Could you check a few things on this model? Use its own coordinates, in mm. Face numbers are marked on the shaded views. A direction names the side the tool comes from. Round coordinates to 2 decimals unless told otherwise and drop trailing zeros. Write each loop counter-clockwise with the first axis right and the second up, starting at its lowest first coordinate (ties: lowest second). Pieces come first, ordered by that corner, then holes. Notation, with made-up numbers: M 52.5,50.25 L 109.5,50.25 A24 ccw 109.5,75.25 Z; hole C 86.5,71.5 d9. An arc over 180 degrees is marked long. One line per item, written item: value. Start each with the question number.
(1) I want a section at A-A on x = 0. Please give me the cut outline in (y, z), and give its area (3 significant figures).
(2) I want a section at B-B on z = 0. Please give me the cut outline in (x, y).
(3) I want a section at D-D on y = 11. Please give me the cut outline in (x, z).
(4) Thinking about a two-plate mould opening in X: for the marked faces 3, 4 and 5, which applies, released by +X, released by -X, zero draft, split by the parting line, or undercut?
(5) If I drill on L1, parallel to X at y = 1.4, z = 0; L2, parallel to Y at x = -1.65, z = -1.35; L3, parallel to Y at x = -0.55, z = 0.25, over which ranges is the centre line in solid material (lowest first)?
(6) I want a section at C-C on y = 8.5. Please give me the cut outline in (x, z), and give its area (3 significant figures).
(7) I'm going to push flat-ended pins straight in: pin 1 Ø1 at (x, z) = (-0.5, 0) entering from -Y; pin 2 Ø2 at (y, z) = (13, 1) entering from -X; pin 3 Ø0.7 at (x, z) = (0, 0) entering from -Y. Where does each tip first touch, or does it pass through?
(8) Which directions (+Z, -Z, +X, -X, +Y, -Y) give clear straight access to the entire face, cutting with the end or side of a thin tool? Please do the marked faces 1 and 2.
```python
from build123d import *

# Parameters (mm, degrees)
SKETCH1_R           = 2.7
BOSS_EXTRUDE1_DEPTH = 2
SKETCH3_R           = 0.95
CUT_EXTRUDE2_DEPTH  = 9.5
SKETCH7_R           = 1.2
CUT_EXTRUDE4_DEPTH  = 2.8
SKETCH2_R           = 1.75
BOSS_EXTRUDE2_DEPTH = 20
FILLET2_R           = 0.5
SKETCH8_R           = 0.95
CUT_EXTRUDE5_DEPTH  = 9.5


with BuildPart() as part:
    # Sketch1 → Boss-Extrude1 (new body)
    with BuildSketch(Plane(origin=(0, 0, 0), x_dir=(1, 0, 0), z_dir=(0, 1, 0))):
        with Locations(Location((0, 0, 0), (0, 0, 270))):
            Circle(SKETCH1_R)
    extrude(amount=BOSS_EXTRUDE1_DEPTH)

    # Sketch3 → Cut-Extrude2 (cut)
    with BuildSketch(Plane.XZ):
        with Locations(Location((0, 0, 0), (0, 0, 270))):
            Circle(SKETCH3_R)
    extrude(amount=-CUT_EXTRUDE2_DEPTH, mode=Mode.SUBTRACT)

    # Sketch7 → Cut-Extrude4 (cut)
    with BuildSketch(Plane.XZ):
        with Locations(Location((0, 0, 0), (0, 0, 270))):
            Circle(SKETCH7_R)
    extrude(amount=-CUT_EXTRUDE4_DEPTH, mode=Mode.SUBTRACT)

    # Sketch2 → Boss-Extrude2 (add)
    with BuildSketch(Plane(origin=(0, 2, 0), x_dir=(1, 0, 0), z_dir=(0, 1, 0))):
        with Locations(Location((0, 0, 0), (0, 0, 270))):
            Circle(SKETCH2_R)
    extrude(amount=BOSS_EXTRUDE2_DEPTH)

    # Fillet2
    fillet2_edges = [part.edges().sort_by_distance(p)[0] for p in [
        (0, 22, -1.75),
    ]]
    fillet(fillet2_edges, radius=FILLET2_R)

    # Sketch8 → Cut-Extrude5 (cut)
    with BuildSketch(Plane.XZ):
        with Locations(Location((0, 0, 0), (0, 0, 270))):
            Circle(SKETCH8_R)
    extrude(amount=-CUT_EXTRUDE5_DEPTH, mode=Mode.SUBTRACT)


solid = part.part
```
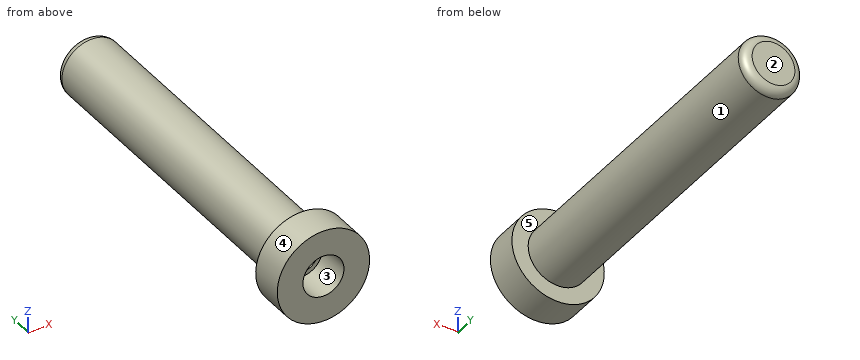
Found:
1. outline: M 0,-2.7 L 2,-2.7 L 2,-1.75 L 21.5,-1.75 A0.5 ccw 22,-1.25 L 22,1.25 A0.5 ccw 21.5,1.75 L 2,1.75 L 2,2.7 L 0,2.7 L 0,1.2 L 2,1.2 L 2,0.95 L 9.5,0.95 L 9.5,-0.95 L 2,-0.95 L 2,-1.2 L 0,-1.2 Z
1. area: 61.6 mm²
2. outline: M -2.7,0 L -1.2,0 L -1.2,2 L -0.95,2 L -0.95,9.5 L 0.95,9.5 L 0.95,2 L 1.2,2 L 1.2,0 L 2.7,0 L 2.7,2 L 1.75,2 L 1.75,21.5 A0.5 ccw 1.25,22 L -1.25,22 A0.5 ccw -1.75,21.5 L -1.75,2 L -2.7,2 Z
3. outline: C 0,0 d3.5
4. face 3: undercut
4. face 4: split by the parting line
4. face 5: zero draft
5. L1: x = -2.7 to -1.2, 1.2 to 2.7
5. L2: y = 0 to 2
5. L3: y = 9.5 to 22
6. outline: C 0,0 d3.5; hole C 0,0 d1.9
6. area: 6.79 mm²
7. pin 1: stops at y = 2
7. pin 2: stops at x = -1.75
7. pin 3: stops at y = 9.5
8. face 1: +Y
8. face 2: +Z, -Z, +X, -X, +Y
